from build123d import *

# Parameters (mm, degrees)
SKETCH2_W                 = 7.5
SKETCH2_H                 = 20
SKETCH2_R                 = 2
BOSS_EXTRUDE1_DEPTH       = 2
SKETCH4_W                 = 21
SKETCH4_H                 = 20
BOSS_EXTRUDE2_DEPTH       = 2
SKETCH5_W                 = 21
SKETCH5_H                 = 46
BOSS_EXTRUDE3_DEPTH       = 2
SKETCH6_W                 = 21
SKETCH6_H                 = 2
BOSS_EXTRUDE4_DEPTH       = 22
SKETCH7_W                 = 6.5
SKETCH7_H                 = 20
SKETCH7_R                 = 2
BOSS_EXTRUDE7_DEPTH       = 2
SKETCH8_W                 = 20
SKETCH8_H                 = 6.5
SKETCH8_R                 = 2
BOSS_EXTRUDE9_DEPTH       = 1.5
SKETCH9_R                 = 2
BOSS_EXTRUDE10_DEPTH      = 1.5
SCALE1_SCALE              = 0.98
SCALE2_SCALE              = 0.98
SCALE3_SCALE              = 1.03
BOSS_EXTRUDE11_DEPTH      = 14
SKETCH13_W                = 1
SKETCH13_H                = 41.546904
BOSS_EXTRUDE12_DEPTH      = 20
SKETCH15_W                = 13.656209454
SKETCH15_H                = 5.440666
CUT_EXTRUDE1_DEPTH        = 20
SKETCH16_W                = 13.65620945
SKETCH16_H                = 5.440666
CUT_EXTRUDE2_DEPTH        = 20
BOSS_EXTRUDE13_DEPTH      = 13.5
SKETCH18_W                = 2.5
SKETCH18_H                = 19.843095219
CUT_EXTRUDE3_DEPTH        = 51.944418
SKETCH19_W                = 1
SKETCH19_H                = 41.546904
BOSS_EXTRUDE14_DEPTH      = 19.78424
CUT_EXTRUDE4_REACH        = 52.944
SKETCH20_W                = 5
SKETCH20_H                = 15
SKETCH21_W                = 10
SKETCH21_H                = 14
CUT_EXTRUDE5_DEPTH        = 19.5
SKETCH22_W                = 5
SKETCH22_H                = 1
BOSS_EXTRUDE15_DEPTH      = 7
BOSS_EXTRUDE15_DEPTH_BACK = 2
SKETCH23_W                = 1.2
SKETCH23_H                = 19.843095219
CUT_EXTRUDE9_DEPTH        = 44


with BuildPart() as part:
    # Sketch2 → Boss-Extrude1 (new body)
    with BuildSketch(Plane(origin=(0, 0, 0), x_dir=(0, 0, -1), z_dir=(1, 0, 0))):
        with Locations((-3.75, -10)):
            Rectangle(SKETCH2_W, SKETCH2_H)
        with Locations((-5, -4.580102725)):
            Circle(SKETCH2_R, mode=Mode.SUBTRACT)
        with Locations((-5, -15)):
            Circle(SKETCH2_R, mode=Mode.SUBTRACT)
    extrude(amount=BOSS_EXTRUDE1_DEPTH)

    # Sketch4 → Boss-Extrude2 (add)
    with BuildSketch(Plane.XY):
        with Locations((10.5, -10)):
            Rectangle(SKETCH4_W, SKETCH4_H)
    extrude(amount=BOSS_EXTRUDE2_DEPTH)

    # Sketch5 → Boss-Extrude3 (add)
    with BuildSketch(Plane(origin=(0, 0, 0), x_dir=(1, 0, 0), z_dir=(0, 1, 0))):
        with Locations((10.5, 21)):
            Rectangle(SKETCH5_W, SKETCH5_H)
    extrude(amount=BOSS_EXTRUDE3_DEPTH)

    # Sketch6 → Boss-Extrude4 (add)
    with BuildSketch(Plane(origin=(0, 2, 0), x_dir=(1, 0, 0), z_dir=(0, 1, 0))):
        with Locations((10.5, 43)):
            Rectangle(SKETCH6_W, SKETCH6_H)
    extrude(amount=-BOSS_EXTRUDE4_DEPTH)

    # Sketch7 → Boss-Extrude7 (add)
    with BuildSketch(Plane.ZY):
        with Locations((-46.25, -10)):
            Rectangle(SKETCH7_W, SKETCH7_H)
        with Locations((-47, -5)):
            Circle(SKETCH7_R, mode=Mode.SUBTRACT)
        with Locations((-47, -15)):
            Circle(SKETCH7_R, mode=Mode.SUBTRACT)
    extrude(amount=-BOSS_EXTRUDE7_DEPTH)

    # Sketch8 → Boss-Extrude9 (add)
    with BuildSketch(Plane.XZ.offset(20)):
        with Locations((11, -46.25)):
            Rectangle(SKETCH8_W, SKETCH8_H)
        with Locations((6, -47)):
            Circle(SKETCH8_R, mode=Mode.SUBTRACT)
        with Locations((16, -47)):
            Circle(SKETCH8_R, mode=Mode.SUBTRACT)
    extrude(amount=-BOSS_EXTRUDE9_DEPTH)

    # Sketch9 → Boss-Extrude10 (add)
    with BuildSketch(Plane.XZ.offset(20)):
        Polygon((21, 2), (21, 7.5), (16, 7.5), (6, 7.5), (2, 7.5), (2, 2), align=None)
        with Locations((6, 5)):
            Circle(SKETCH9_R, mode=Mode.SUBTRACT)
        with Locations((16, 5)):
            Circle(SKETCH9_R, mode=Mode.SUBTRACT)
    extrude(amount=-BOSS_EXTRUDE10_DEPTH)


with BuildPart() as part_1:
    # Scale1: scaled about (9.7960723, -5.455619142, -21)
    add(part.part.scale(SCALE1_SCALE).moved(Location((0.195921446, -0.109112383, -0.42))))


with BuildPart() as part_2:
    # Scale2: scaled about (9.7960723, -5.455619142, -21)
    add(part_1.part.scale(SCALE2_SCALE).moved(Location((0.195921446, -0.109112383, -0.42))))


with BuildPart() as part_3:
    # Scale3: scaled about (9.7960723, -5.455619142, -21)
    add(part_2.part.scale(SCALE3_SCALE).moved(Location((-0.293882169, 0.163668574, 0.63))))

    # Sketch11 → Boss-Extrude11 (add)
    with BuildSketch(Plane(origin=(20.879132028, 0, 0), x_dir=(0, 0, -1), z_dir=(1, 0, 0))):
        Polygon((-1.751876, 1.919568781), (43.751876, 1.919568781), (43.751876, -18.359277219), (49.192542, -18.359277219), (49.192542, -19.843095219), (41.773452, -19.843095219), (41.773452, -0.058855219), (0.226548, -0.058855219), (0.226548, -19.843095219), (-7.192542, -19.843095219), (-7.192542, -18.359277219), (-1.751876, -18.359277219), align=None)
    extrude(amount=BOSS_EXTRUDE11_DEPTH)

    # Sketch13 → Boss-Extrude12 (add)
    with BuildSketch(Plane(origin=(0, -0.058855219, 0), x_dir=(-1, 0, 0), z_dir=(0, -1, 0))):
        with Locations((-34.379132028, 21)):
            Rectangle(SKETCH13_W, SKETCH13_H)
    extrude(amount=BOSS_EXTRUDE12_DEPTH)

    # Sketch15 → Cut-Extrude1 (cut)
    with BuildSketch(Plane(origin=(0, -18.359277219, 0), x_dir=(1, 0, 0), z_dir=(0, 1, 0))):
        with Locations((28.051027301, 46.472209)):
            Rectangle(SKETCH15_W, SKETCH15_H)
    extrude(amount=-CUT_EXTRUDE1_DEPTH, mode=Mode.SUBTRACT)

    # Sketch16 → Cut-Extrude2 (cut)
    with BuildSketch(Plane(origin=(0, -18.359277219, 0), x_dir=(1, 0, 0), z_dir=(0, 1, 0))):
        with Locations((28.051027303, -4.472209)):
            Rectangle(SKETCH16_W, SKETCH16_H)
    extrude(amount=-CUT_EXTRUDE2_DEPTH, mode=Mode.SUBTRACT)

    # Sketch17 → Boss-Extrude13 (add)
    with BuildSketch(Plane.ZY.offset(-0.105680028)):
        Polygon((1.751876, 1.919568781), (-43.751876, 1.919568781), (-43.751876, -0.058855219), (-43.751876, -19.843095219), (-41.773452, -19.843095219), (-41.773452, -0.058855219), (-0.226548, -0.058855219), (-0.226548, -19.843095219), (1.751876, -19.843095219), (1.751876, -0.058855219), align=None)
    extrude(amount=BOSS_EXTRUDE13_DEPTH)

    # Sketch18 → Cut-Extrude3 (cut, through all)
    with BuildSketch(Plane.XY.offset(1.751876)):
        with Locations((-1.144319972, -9.92154761)):
            Rectangle(SKETCH18_W, SKETCH18_H)
    extrude(amount=-CUT_EXTRUDE3_DEPTH, mode=Mode.SUBTRACT)

    # Sketch19 → Boss-Extrude14 (add)
    with BuildSketch(Plane.XZ.offset(0.058855219)):
        with Locations((-12.894319972, -21)):
            Rectangle(SKETCH19_W, SKETCH19_H)
    extrude(amount=BOSS_EXTRUDE14_DEPTH)

    # Sketch20 → Cut-Extrude4 (cut, up to next)
    with BuildSketch(Plane.XY.offset(1.751876), mode=Mode.PRIVATE) as cut_extrude4_sk1:
        with Locations((26.584104028, -12.343095219)):
            Rectangle(SKETCH20_W, SKETCH20_H)
    cut_extrude4_tool1 = extrude(cut_extrude4_sk1.sketch, amount=-CUT_EXTRUDE4_REACH, mode=Mode.PRIVATE) & part_3.part
    add(cut_extrude4_tool1.solids().sort_by_distance((26.584104, -12.343095, 1.751876))[0], mode=Mode.SUBTRACT)

    # Sketch21 → Cut-Extrude5 (cut)
    with BuildSketch(Plane.ZY.offset(13.394319972)):
        with Locations((-9.248124, -12.843095219)):
            Rectangle(SKETCH21_W, SKETCH21_H)
    extrude(amount=-CUT_EXTRUDE5_DEPTH, mode=Mode.SUBTRACT)

    # Sketch22 → Boss-Extrude15 (add, two sides)
    with BuildSketch(Plane.XY.offset(1.751876)) as boss_extrude15_sk:
        with Locations((26.584104028, -4.343095219)):
            Rectangle(SKETCH22_W, SKETCH22_H)
    extrude(amount=BOSS_EXTRUDE15_DEPTH)
    extrude(boss_extrude15_sk.sketch, amount=-BOSS_EXTRUDE15_DEPTH_BACK)

    # Sketch23 → Cut-Extrude9 (cut)
    with BuildSketch(Plane(origin=(0, 0, -43.751876), x_dir=(-1, 0, 0), z_dir=(0, 0, -1))):
        with Locations((2.994319972, -9.92154761)):
            Rectangle(SKETCH23_W, SKETCH23_H)
    extrude(amount=-CUT_EXTRUDE9_DEPTH, mode=Mode.SUBTRACT)


solid = part_3.part
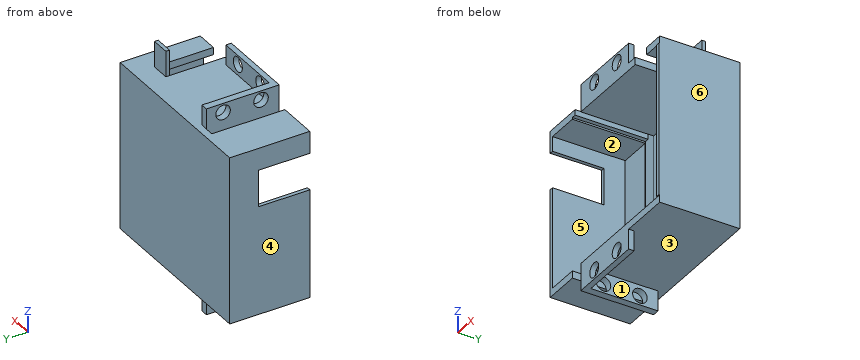
The model under review builds one solid part; all positions refer to its coordinate system, in mm. Face numbers are marked on the shaded views. A direction names the side the tool comes from. Coordinates: 2 decimals unless noted, no trailing zeros. Write each loop counter-clockwise with the first axis right and the second up, starting at its lowest first coordinate (ties: lowest second). Pieces come first, ordered by that corner, then holes. Notation, with made-up numbers: M 35.25,51.5 L 76.25,51.5 A18 ccw 76.25,82.5 Z; hole C 39,76.25 d7. An arc over 180 degrees is marked long. Put each result on its own line as item: value.
1) Add section C-C on z = -28. Give the boundary of the cut face in (x, y).
Computed:
outline: M -13.39,-19.84 L -12.39,-19.84 L -12.39,-0.06 L -3.59,-0.06 L -3.59,0 L 0.11,0 L 0.11,-0.06 L 33.88,-0.06 L 33.88,-20.06 L 34.88,-20.06 L 34.88,1.92 L -13.39,1.92 Z
2) Add section A-A on y = -7.75. State how many separate pieces and enclosed holes the cut face has, then the cut area to 3 significant figures.
Computed:
separate pieces: 4
enclosed holes: 0
area: 263 mm2
3) Wall thickness on probe 1 along X at (y, z) = (-13.5, -42.5); probe 2 along Z at (x, y) = (32, -0.25); probe 3 along X at (y, z) = (-19, -34): over which ranges is each line inside the solid? List them lowest first. Write a range as [from, to].
Computed:
probe 1: x = [-13.39, -3.59], [0.11, 34.88]
probe 2: z = [-43.75, -41.77], [-0.23, 1.75]
probe 3: x = [-13.39, -12.39], [33.88, 34.88]
4) Add section D-D on x = -1. Give the boundary of the cut face in (y, z), then the cut area to 3 significant figures.
Computed:
outline: M 0,-43.75 L 1.92,-43.75 L 1.92,1.75 L 0,1.75 Z
area: 87.3 mm2
5) Clearance check with flat-ended pins moving along their axes: pin 1 Ø4 at (y, z) = (-8, -10.5) entering from -X; pin 2 Ø6 at (x, y) = (11, -13) entering from +Z; pin 3 Ø4 at (x, z) = (9.5, -2.5) entering from -Y. State where each tip first meets the part, or that it passes through.
Computed:
pin 1: stops at x = 33.88
pin 2: stops at z = 1.75
pin 3: stops at y = -0.06
6) Draft analysis for pull direction X (two halves, no side actions). For the marked faces 4, 5 and 6, state which applies: released by +X, released by -X, zero draft, split by the parting line, or undercut.
Computed:
face 4: released by -X
face 5: undercut
face 6: released by +X
7) Add section B-B on x = 15. Give the boundary of the cut face in (y, z).
Computed:
outline: M -19.84,-49.19 L -18.36,-49.19 L -18.36,-48.46 L -19.84,-48.46 Z; M -19.84,-44.97 L -18.36,-44.97 L -18.36,-43.75 L 1.92,-43.75 L 1.92,1.75 L -18.36,1.75 L -18.36,2.97 L -19.84,2.97 L -19.84,-0.23 L -0.06,-0.23 L -0.06,-41.77 L -19.84,-41.77 Z; M -19.84,6.46 L -18.36,6.46 L -18.36,7.19 L -19.84,7.19 Z
8) For the marked faces 1, 2 and 3, list the 3-axis set-ups (+Z, -Z, +X, -X, +Y, -Y) from which the entire face can be reached by the end or side of a thin tool; tool diameter is ignored.
Computed:
face 1: -Z, +X, +Y
face 2: -Y
face 3: -Z, +Y
